Geometry check sheet. Reference: the model listing, model coordinates, mm. Face numbers are marked on the shaded views. A direction names the side the tool comes from. Round coordinates to 2 decimals unless told otherwise and drop trailing zeros. Order: outer loops, then holes, each group sorted by start corner. A loop starts at its lowest first (then second) coordinate and runs counter-clockwise, first axis right, second up. Notation, with made-up numbers: (21, 26) - (69, 26) arc R18 cw to (69, 39) - close; hole circle Ø10 at (45, -15). An arc over 180 degrees is marked (long way). Write each question's results on one line, items separated by ' | '.
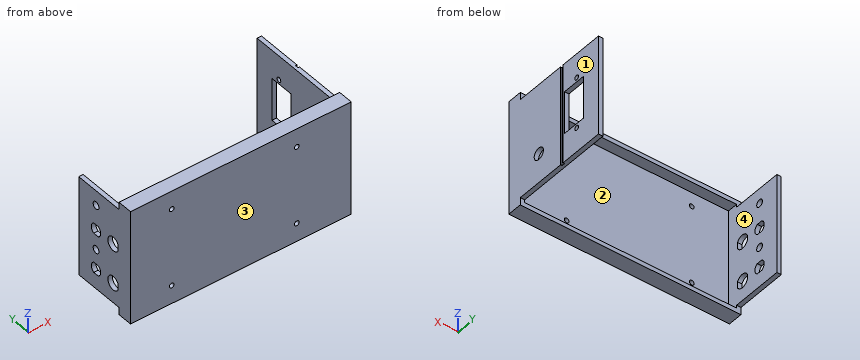
Autodesk Inventor part; units mm, degrees
ref_plane "YZ Plane" through (0, 0, 0) normal (1, 0, 0) x (0, 1, 0)
ref_plane "XZ Plane" through (0, 0, 0) normal (0, 1, 0) x (-1, 0, 0)
ref_plane "XY Plane" through (0, 0, 0) normal (0, 0, 1) x (1, 0, 0)
sketch "Sketch1" plane through (0, 0, 0) normal (0, 1, 0) x (-1, 0, 0)
  line L0 (-75, -39) -> (75, -39)
  line L1 (75, -39) -> (75, 39)
  line L2 (75, 39) -> (-75, 39)
  line L3 (-75, 39) -> (-75, -39)
  line L4 (-75, -39) -> (75, 39) construction
  line L5 (75, -39) -> (-75, 39) construction
  point P0 (0, 0)
  dimension "d0" = 150
  dimension "d1" = 78
extrude "Extrusion1" add sketch "Sketch1" along normal blind 45
sketch "Sketch4" plane through (75, 0, 39) normal (1, 0, 0) x (0, 0, -1)
  line L0 (78, 45) -> (0, 45)
  line L1 (0, 45) -> (5, 45)
  line L2 (5, 45) -> (5, 10)
  line L3 (5, 10) -> (0, 10)
  line L4 (0, 10) -> (0, 45)
  line L5 (78, 45) -> (73, 45)
  line L6 (73, 45) -> (73, 10)
  line L7 (73, 10) -> (78, 10)
  line L8 (78, 10) -> (78, 45)
  point P0 (39, 0)
  dimension "d14" = 5
  dimension "d15" = 35
  dimension "d16" = 5
  dimension "d17" = 35
extrude "Extrusion4" cut sketch "Sketch4" against normal blind 150
sketch "Sketch5" plane through (0, 45, 0) normal (0, 1, 0) x (1, 0, 0)
  line L0 (72, 36) -> (-72, 36)
  line L1 (-72, 36) -> (-72, -36)
  line L2 (-72, -36) -> (72, -36)
  line L3 (72, -36) -> (72, 36)
  line L4 (72, 36) -> (-72, -36) construction
  line L5 (-72, 36) -> (72, -36) construction
  point P0 (0, 0)
  dimension "d20" = 144
  dimension "d21" = 72
extrude "Extrusion5" cut sketch "Sketch5" against normal blind 42
sketch "Sketch6" plane through (75, 0, 39) normal (1, 0, 0) x (0, 0, -1)
  circle A0 centre (53, 26.1062) radius 4
  line L0 (73, 10) -> (73, 45)
  circle A1 centre (25, 27.5) radius 10.75
  line L1 (5, 78) -> (5, 10)
  point P0 (39, 0)
  point P1 (5, 45)
  dimension "d25" = 8
  dimension "d33" = 20
  dimension "d67" = 21.5
  dimension "d68" = 20
sketch "Sketch7" plane through (-75, 0, -39) normal (-1, 0, 0) x (0, 0, 1)
  line L0 (22.15, 28.0506) -> (22.15, 31.9494)
  line L1 (15.05, 31.9494) -> (15.05, 28.0506)
  line L2 (15.05, 28.0506) -> (22.15, 31.9494) construction
  line L3 (22.15, 28.0506) -> (15.05, 31.9494) construction
  arc A0 (22.15, 31.9494) -> (15.05, 31.9494) centre (18.6, 30) ccw
  arc A1 (15.05, 28.0506) -> (22.15, 28.0506) centre (18.6, 30) ccw
  line L4 (18.6, 30) -> (18, 30) construction
  line L5 (0, 0) -> (78, 0)
  line L6 (5, 45) -> (5, 10)
  arc A2 (20.8062, 10.85) -> (16.3938, 10.85) centre (18.6, 15) ccw
  line L7 (16.3938, 10.85) -> (20.8062, 10.85)
  circle A3 centre (32.2, 30) radius 2.5
  line L8 (49.35, 28.0506) -> (49.35, 31.9494)
  line L9 (42.25, 31.9494) -> (42.25, 28.0506)
  line L10 (42.25, 28.0506) -> (49.35, 31.9494) construction
  line L11 (49.35, 28.0506) -> (42.25, 31.9494) construction
  arc A4 (49.35, 31.9494) -> (42.25, 31.9494) centre (45.8, 30) ccw
  arc A5 (42.25, 28.0506) -> (49.35, 28.0506) centre (45.8, 30) ccw
  line L12 (45.8, 30) -> (41.8, 30) construction
  line L13 (43.5938, 10.85) -> (48.0062, 10.85)
  arc A6 (48.0062, 10.85) -> (43.5938, 10.85) centre (45.8, 15) ccw
  circle A7 centre (62.8, 30) radius 2.5
  point P0 (39, 0)
  point P1 (18.6, 30)
  point P2 (18.6, 30)
  dimension "d36" = 7.1
  dimension "d37" = 4.05
  dimension "d77" = 30
  dimension "d81" = 13.6
  dimension "d85" = 9.4
  dimension "d86" = 4.15
  dimension "d87" = 15
  dimension "d88" = 5
  dimension "d89" = 13.6
  dimension "d90" = 7.1
  dimension "d91" = 4.05
  dimension "d92" = 9.4
  dimension "d93" = 4.15
  dimension "d94" = 15
  dimension "d95" = 5
  dimension "d96" = 17
  dimension "d97" = 13.6
sketch "Sketch8" plane through (0, 3, 0) normal (0, 1, 0) x (1, 0, 0)
  line L0 (-47, -26.5) -> (38, -26.5)
  line L1 (38, -26.5) -> (38, 26.5)
  line L2 (38, 26.5) -> (-47, 26.5)
  line L3 (-47, 26.5) -> (-47, -26.5)
  line L4 (-47, -26.5) -> (38, 26.5) construction
  line L5 (38, -26.5) -> (-47, 26.5) construction
  circle A0 centre (38, 26.5) radius 1.6
  circle A1 centre (38, -26.5) radius 1.6
  circle A2 centre (-47, -26.5) radius 1.6
  circle A3 centre (-47, 26.5) radius 1.6
  line L6 (-72, -34) -> (-72, 34)
  point P0 (-4.5, 0)
  dimension "d42" = 85
  dimension "d43" = 53
  dimension "d44" = 3.2
  dimension "d45" = 3.2
  dimension "d46" = 3.2
  dimension "d47" = 3.2
  dimension "d51" = 25
extrude "Extrusion8" cut sketch "Sketch8" against normal blind 3 contours L3 A2 L0 | L0 A2 L3 | A1 L1 L0 | L0 L1 A1 | A3 L2 L3 | L3 L2 A3 | A0 L2 L1 | L1 L2 A0
sketch "Sketch9" plane through (0, 45, 0) normal (0, 1, 0) x (1, 0, 0)
  line L0 (75, -34) -> (72, -34)
  line L1 (75, 39) -> (75, 34)
  line L2 (72, -34) -> (75, -34)
  line L3 (75, -34) -> (75, 34)
  line L4 (75, 34) -> (72, 34)
  line L5 (72, 34) -> (72, -34)
  point P0 (0, 0)
extrude "Extrusion9" add sketch "Sketch9" along normal blind 33
sketch "Sketch10" plane through (75, 0, 39) normal (1, 0, 0) x (0, 0, -1)
  line L0 (53.5, 65) -> (24.5, 65)
  line L1 (24.5, 65) -> (24.5, 48.5)
  line L2 (24.5, 48.5) -> (53.5, 48.5)
  line L3 (53.5, 48.5) -> (53.5, 65)
  line L4 (53.5, 65) -> (24.5, 48.5) construction
  line L5 (24.5, 65) -> (53.5, 48.5) construction
  line L6 (61.5, 65) -> (16.5, 65)
  line L7 (16.5, 65) -> (16.5, 48.5)
  line L8 (16.5, 48.5) -> (61.5, 48.5)
  line L9 (61.5, 48.5) -> (61.5, 65)
  line L10 (61.5, 65) -> (16.5, 48.5) construction
  line L11 (16.5, 65) -> (61.5, 48.5) construction
  line L12 (39, 48.5) -> (39, 65) construction
  line L13 (5, 78) -> (73, 78)
  line L14 (5, 78) -> (5, 10)
  circle A0 centre (21.5, 59) radius 1.6
  line L15 (39, 65) -> (39, 48.5)
  circle A1 centre (56.5, 59) radius 1.6
  point P0 (39, 0)
  point P1 (39, 56.75)
  point P2 (39, 56.75)
  dimension "d54" = 29
  dimension "d55" = 16.5
  dimension "d56" = 45
  dimension "d59" = 13
  dimension "d60" = 34
  dimension "d61" = 3.2
  dimension "d62" = 5
  dimension "d74" = 10.5
extrude "Extrusion10" cut sketch "Sketch10" against normal blind 3 contours L3 L2 L15 L0 | L15 L2 L1 L0 | A0 | A1
sketch "Sketch11" plane through (75, 0, 39) normal (1, 0, 0) x (0, 0, -1)
  point P0 (39, 0)
sketch "Sketch12" plane through (75, 0, 39) normal (1, 0, 0) x (0, 0, -1)
  line L0 (5, 78) -> (5, 10)
  line L1 (5, 45) -> (73, 45)
  line L2 (73, 45) -> (73, 47)
  line L3 (73, 47) -> (5, 47)
  line L4 (5, 47) -> (5, 45)
  line L5 (0, 0) -> (78, 0)
  line L6 (73, 10) -> (73, 78)
  point P0 (39, 0)
  dimension "d69" = 45
  dimension "d70" = 2
extrude "Extrusion12" cut sketch "Sketch12" against normal blind 1
extrude "Extrusion13" cut sketch "Sketch6" against normal blind 10 contours A0
extrude "Extrusion14" cut sketch "Sketch7" against normal blind 10
properties part number "box"
(1) Material ranges on line 1 (Z direction, x = 38, y = 1.55); line 2 (X direction, y = 21, z = -4.5); line 3 (Y direction, x = 72.9, z = 17.5), recorded low to high.
Answers follow:
line 1: -39 to -28.1, -24.9 to 24.9, 28.1 to 39 | line 2: -75 to -72, 72 to 75 | line 3: 0 to 57.4, 60.6 to 78
(2) Section check A-A (y = 15). Record the cut outline in (x, z), then the cut area to 3 significant figures.
Answers follow:
outline: (-75, -34) - (-72, -34) - (-72, -25.1) - (-75, -25.1) - close; (-75, -15.7) - (-72, -15.7) - (-72, 2.1) - (-75, 2.1) - close; (-75, 11.5) - (-72, 11.5) - (-72, 34) - (-75, 34) - close; (72, -34) - (75, -34) - (75, 34) - (72, 34) - close | area: 352 mm²
(3) Access from +Z, -Z, +X, -X, +Y, -Y to the whole of each face (thin tool, end or side, straight path). Record for the marked faces 3 and 4.
Answers follow:
face 3: +Z, -Z, +X, -X, -Y | face 4: +Y
(4) Section check D-D (y = 42). Record the cut outline in (x, z), then the cut area to 3 significant figures.
Answers follow:
outline: (-75, -34) - (-72, -34) - (-72, 34) - (-75, 34) - close; (72, -34) - (75, -34) - (75, 34) - (72, 34) - close | area: 408 mm²
(5) Section check C-C (z = 17.5). Record the cut outline in (x, y).
Answers follow:
outline: (-75, 0) - (75, 0) - (75, 45) - (74, 45) - (74, 47) - (75, 47) - (75, 57.4) - (72, 57.4) - (72, 3) - (-72, 3) - (-72, 45) - (-75, 45) - close; (72, 60.6) - (75, 60.6) - (75, 78) - (72, 78) - close
(6) Depth check by flat-ended pin: pin 1 Ø3 at (x, z) = (38, -26.5) entering from +Y; pin 2 Ø6 at (x, z) = (-6, 16) entering from +Y; pin 3 Ø0.9 at (x, y) = (73.5, 60) entering from -Z; pin 4 Ø2.5 at (x, y) = (-73.5, 26.5) entering from +Z. Enter the tip coordinate at first touch or a pass-through.
Answers follow:
pin 1: through | pin 2: y = 3 | pin 3: z = -34 | pin 4: z = 34
(7) Section check B-B (x = 38). Record the cut outline in (y, z).
Answers follow:
outline: (0, -39) - (10, -39) - (10, -36) - (3, -36) - (3, -28.1) - (0, -28.1) - close; (0, -24.9) - (3, -24.9) - (3, 24.9) - (0, 24.9) - close; (0, 28.1) - (3, 28.1) - (3, 36) - (10, 36) - (10, 39) - (0, 39) - close
(8) Draft check along Z on the marked faces 1 and 2. Enter one of: released by +Z, released by -Z, zero draft, split by the parting line, or undercut.
Answers follow:
face 1: zero draft | face 2: undercut
